For this review, take the finished solid that the model builds, in its own axes (mm). A direction names the side the tool comes from. Round coordinates to 2 decimals unless told otherwise and drop trailing zeros. Order: outer loops, then holes, each group sorted by start corner. A loop starts at its lowest first (then second) coordinate and runs counter-clockwise, first axis right, second up. Notation, with made-up numbers: (28, 23) -> (62, 23) arc R34 cw to (62, 57) -> close; hole circle Ø2 at (63.25, -11). An arc over 180 degrees is marked (long way). Answer in a Markdown table with one row per item.
```python
from build123d import *

# Parameters (mm, degrees)
BOSS_EXTRUDE1_DEPTH = 300
SKETCH3_W           = 39
SKETCH3_H           = 95.8
CUT_EXTRUDE2_DEPTH  = 15
SKETCH5_W           = 10
SKETCH5_H           = 40
CUT_EXTRUDE3_DEPTH  = 10


with BuildPart() as part:
    # Sketch2 → Boss-Extrude1 (new body)
    with BuildSketch(Plane.XY):
        Polygon((68.204834584, -44.523707756), (68.204834584, -38.523707756), (-31.795165416, -21.430394722), (-31.795165416, -27.430394722), align=None)
    extrude(amount=BOSS_EXTRUDE1_DEPTH)

    # Sketch3 → Cut-Extrude2 (cut)
    with BuildSketch(Plane(origin=(-4.461794575, -26.102573363, 0), x_dir=(0.9857034690888548, -0.1684893795649959, 0), z_dir=(0.16848937956499588, 0.9857034690888546, 0))):
        with Locations((22.995383369, -147.9)):
            Rectangle(SKETCH3_W, SKETCH3_H)
    extrude(amount=-CUT_EXTRUDE2_DEPTH, mode=Mode.SUBTRACT)

    # Sketch5 → Cut-Extrude3 (cut)
    with BuildSketch(Plane(origin=(-4.461794575, -26.102573363, 0), x_dir=(0.9857034690888548, -0.16848937956499582, 0), z_dir=(0.16848937956499585, 0.9857034690888549, 0))):
        with Locations((55.720577677, -47.61631705)):
            Rectangle(SKETCH5_W, SKETCH5_H)
    extrude(amount=-CUT_EXTRUDE3_DEPTH, mode=Mode.SUBTRACT)


solid = part.part
```
Q1. Clearance check with flat-ended pins moving along their axes: pin 1 Ø6 at (x, z) = (5, 253.5) entering from +Y; pin 2 Ø5 at (x, z) = (-17.5, 258.5) entering from -Y; pin 3 Ø3 at (x, z) = (-7, 116.5) entering from +Y. State where each tip first meets the part, or that it passes through.
Answer key:
| item | result |
|---|---|
| pin 1 | stops at y = -27.21 |
| pin 2 | stops at y = -30.3 |
| pin 3 | stops at y = -25.41 |
Q2. To check wall thickness, follow probe 1 along Z at (x, y) = (33, -33.25); probe 2 along Z at (x, y) = (46.5, -37.5); probe 3 along Y at (x, z) = (-27, 44). State the ranges of each line that lie inside material, in increasing order.
Answer key:
| item | result |
|---|---|
| probe 1 | z = 0 to 100, 195.8 to 300 |
| probe 2 | z = 0 to 27.62, 67.62 to 300 |
| probe 3 | y = -28.25 to -22.25 |
Q3. Tool access review of faces 5 (the face through (45.042, -37.522, 47.896)), 6 (the face through (54.9, -39.2, 47.9)), 7 (the face through (-1.51, -29.57, 148.57)), 8 (the face through (-4.72, -32.06, 147.9)), 9 (the face through (36.935, -36.137, 148.571)): name each direction out of +Z, -Z, +X, -X, +Y, -Y from which nothing blocks a thin tool from reaching the whole face with its end or side.
Answer key:
| item | result |
|---|---|
| face 5 | -Y |
| face 6 | +Y |
| face 7 | +X, -Y |
| face 8 | +Z, -Z, -X, -Y |
| face 9 | -X, +Y |
Q4. Take a section at B-B, the plane x = 32.5. Write out the cut boundary in (y, z), then the cut area to 3 significant figures.
Answer key:
| item | result |
|---|---|
| outline | (-38.42, 0) -> (-32.42, 0) -> (-32.42, 100) -> (-38.42, 100) -> close; (-38.42, 195.8) -> (-32.42, 195.8) -> (-32.42, 300) -> (-38.42, 300) -> close |
| area | 1,230 mm^2 |
Q5. Take a section at A-A, the plane z = 168.5. Write out the cut boundary in (x, y).
Answer key:
| item | result |
|---|---|
| outline | (-31.8, -27.43) -> (-2.01, -32.52) -> (-1.02, -26.69) -> (-31.8, -21.43) -> close; (36.43, -39.09) -> (68.2, -44.52) -> (68.2, -38.52) -> (37.43, -33.26) -> close |
Q6. Take a section at D-D, the plane x = -23. Write out the cut boundary in (y, z), then the cut area to 3 significant figures.
Answer key:
| item | result |
|---|---|
| outline | (-28.93, 0) -> (-22.93, 0) -> (-22.93, 300) -> (-28.93, 300) -> close |
| area | 1,800 mm^2 |
Q7. Take a section at C-C, the plane z = 276. Write out the cut boundary in (x, y), then the cut area to 3 significant figures.
Answer key:
| item | result |
|---|---|
| outline | (-31.8, -27.43) -> (68.2, -44.52) -> (68.2, -38.52) -> (-31.8, -21.43) -> close |
| area | 600 mm^2 |
Q8. The part is to be moulded in two halves that separate along Z. For faces 1 (the face through (17, -33, 100)), 2 (the face through (-31.795, -24, 148)), 3 (the face through (18, -34, 0)), 4 (the face through (18, -34, 300)), say which applies: +Z half, -Z half, draft (parallel to the pull), parting line (faces both ways), or undercut.
Answer key:
| item | result |
|---|---|
| face 1 | undercut |
| face 2 | draft |
| face 3 | -Z half |
| face 4 | +Z half |
